```python
from build123d import *

# Parameters (mm, degrees)
SKETCH_1_R      = 10
EXTRUDE_1_DEPTH = 21.5
SKETCH_2_R      = 9
EXTRUDE_2_DEPTH = 16
CHAMFER_1_SIZE  = 0.5


with BuildPart() as part:
    # 草图1 → 凸台-拉伸1 (new body)
    with BuildSketch(Plane.XY):
        Circle(SKETCH_1_R)
    extrude(amount=EXTRUDE_1_DEPTH)

    # 草图2 → 凸台-拉伸2 (add)
    with BuildSketch(Plane.XY.offset(21.5)):
        Circle(SKETCH_2_R)
    extrude(amount=EXTRUDE_2_DEPTH)

    # 倒角1
    chamfer_1_edges = [part.edges().sort_by_distance(p)[0] for p in [
        (-10, 0, 0),
        (-10, 0, 21.5),
        (-9, 0, 37.5),
    ]]
    chamfer(chamfer_1_edges, length=CHAMFER_1_SIZE)


solid = part.part
```
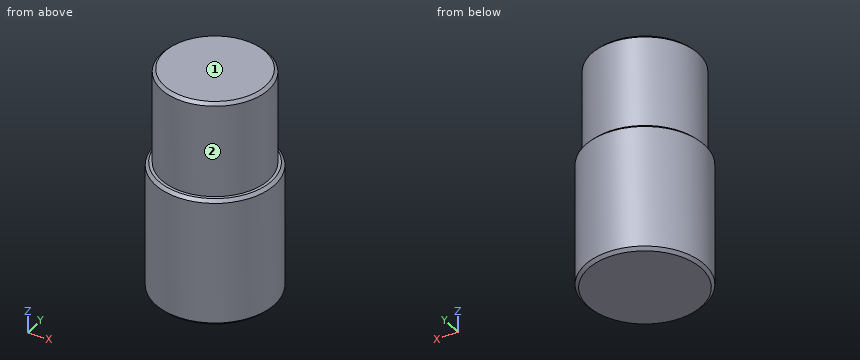
Geometry check sheet. Reference: the model listing, model coordinates, mm. Face numbers are marked on the shaded views. A direction names the side the tool comes from. Coordinates: 2 decimals unless noted, no trailing zeros. Write each loop counter-clockwise with the first axis right and the second up, starting at its lowest first coordinate (ties: lowest second). Pieces come first, ordered by that corner, then holes. Notation, with made-up numbers: M 22,-6.75 L 63,-6.75 A24 cw 63,21.25 Z; hole C 66.5,4 d4. An arc over 180 degrees is marked long. Use one line per item in the form item = value. Start each with the question number.
1) Set-up check for the marked faces 1 and 2: record each of +Z, -Z, +X, -X, +Y, -Y from which the full face is reachable in a straight line by a thin tool's end or side.
2) Section check D-D on z = 23. Enter the section's corners in (x, y), and give its area (3 significant figures).
3) Section check A-A on x = 0. Enter the section's corners in (y, z).
4) Section check C-C on z = 11.5. Enter the section's corners in (x, y), and give its area (3 significant figures).
5) Thickness scan on probe 1 along X at (y, z) = (5.25, 7); probe 2 along Y at (x, z) = (0, 20); probe 3 along Y at (x, z) = (-8.25, 14). Record the ranges inside material, lowest first. Write a range as from..to.
6) Go/stop test with flat-tipped pins: pin 1 Ø3 at (x, z) = (-0.5, 31.5) entering from -Y; pin 2 Ø10 at (y, z) = (2.5, 12.5) entering from -X; pin 3 Ø2 at (x, z) = (2.5, 30) entering from +Y; pin 4 Ø6 at (y, z) = (3.5, 33.5) entering from -X. Record where each tip stops, or that it passes through.
Responses:
q1.face_1 = +Z, +X, -X, +Y, -Y
q1.face_2 = +Z
q2.outline = C 0,0 d18
q2.area = 254 mm2
q3.outline = M -10,0.5 L -9.5,0 L 9.5,0 L 10,0.5 L 10,21 L 9.5,21.5 L 9,21.5 L 9,37 L 8.5,37.5 L -8.5,37.5 L -9,37 L -9,21.5 L -9.5,21.5 L -10,21 Z
q4.outline = C 0,0 d20
q4.area = 314 mm2
q5.probe_1 = -8.51..8.51
q5.probe_2 = -10..10
q5.probe_3 = -5.65..5.65
q6.pin_1 = -9
q6.pin_2 = -10
q6.pin_3 = 8.87
q6.pin_4 = -8.99
